Build history of the part. All positions in model axes, mm. A direction names the side the tool comes from. Round coordinates to 2 decimals unless told otherwise and drop trailing zeros. Write each loop counter-clockwise with the first axis right and the second up, starting at its lowest first coordinate (ties: lowest second). Pieces come first, ordered by that corner, then holes.
1) Saw through at C-C (z = 23.5). Write the cut outline in (x, y).
2) Saw through at D-D (y = 7.5). Write the cut outline in (x, z).
3) Which spindle directions (+Z, -Z, +X, -X, +Y, -Y) get a long thin tool onto all of the face, cutting with end or side? Do faces 1 (the flat face through (4.83, -8.21, 5.48)), 2 (the flat face through (-6.5, 0.2, 11.112)). Say none if no direction does.
4) Wall check: probe 1 along Z at (x, y) = (-3.25, -8); probe 2 along X at (y, z) = (-0.25, 15.5); probe 3 along Y at (x, z) = (3.25, 14). Give the ranges that are in metal, low to high.
5) Flat gauge pins, fed straight in: pin 1 (8 mm diameter, centred on x = 6.5, z = 18.5, fed in from -Y); pin 2 (10 mm diameter, centred on y = 7, z = 17.5, fed in from +X); pin 3 (12 mm diameter, centred on y = -7.5, z = 21, fed in from -X). Where does each tip first touch, or does it go through?
6) Saw through at B-B (x = 2). Write the cut outline in (y, z), plus the area to 3 significant figures.
Autodesk Inventor part; units mm, degrees
ref_plane "YZ Plane" through (0, 0, 0) normal (1, 0, 0) x (0, 1, 0)
ref_plane "XZ Plane" through (0, 0, 0) normal (0, 1, 0) x (-1, 0, 0)
ref_plane "XY Plane" through (0, 0, 0) normal (0, 0, 1) x (1, 0, 0)
sketch "Sketch1" plane through (0, 0, 0) normal (0, 0, 1) x (1, 0, 0)
  line L0 (-9.525, 5.4993) -> (0, 10.9985)
  line L1 (0, 10.9985) -> (9.525, 5.4993)
  line L2 (9.525, 5.4993) -> (9.525, -5.4993)
  line L3 (9.525, -5.4993) -> (0, -10.9985)
  line L4 (0, -10.9985) -> (-9.525, -5.4993)
  line L5 (-9.525, -5.4993) -> (-9.525, 5.4993)
  point P0 (0, 0)
  point P1 (0, 0)
  dimension "d0" = 19.05
extrude "Extrusion1" add sketch "Sketch1" along normal blind 11.1125
sketch "Sketch2" plane through (0, 0, 11.1125) normal (0, 0, 1) x (1, 0, 0)
  circle A0 centre (0, 0) radius 6.35
  point P0 (0, 0)
  dimension "d3" = 12.7
extrude "Extrusion2" add sketch "Sketch2" along normal blind 25.4
properties part number "short half-inch hex bolt" material "Steel"
Evaluation:
1. outline: circle Ø12.7 at (0, 0)
2. outline: (-6.06, 0) - (6.06, 0) - (6.06, 11.11) - (-6.06, 11.11) - close
3. face 1: +Z, -Z, +X, -Y
3. face 2: +Z
4. probe 1: z = 0 to 11.11
4. probe 2: x = -6.35 to 6.35
4. probe 3: y = -5.46 to 5.46
5. pin 1: stops at y = -5.84
5. pin 2: stops at x = 6.03
5. pin 3: stops at x = -6.17
6. outline: (-9.84, 0) - (9.84, 0) - (9.84, 11.11) - (6.03, 11.11) - (6.03, 36.51) - (-6.03, 36.51) - (-6.03, 11.11) - (-9.84, 11.11) - close
6. area: 525 mm2
